Source: three-view drawing plus pictorial views. Frame: mm from the lowest corner of the part. Round coordinates to 2 decimals unless told otherwise and drop trailing zeros. Loops run counter-clockwise (first coordinate to the right, second up) from the corner with the lowest first, then second, coordinate; pieces in that order, holes last. Notation, with made-up numbers: (51, 25) -> (110, 25) arc R27 ccw to (110, 47) -> close; hole circle Ø2 at (54, -13.75). An arc over 180 degrees is marked (long way). One line per question, with ' | ' between items. Start each with the question number.
Q1. Cut plane D-D on x = 5.5. Return loops of the section in (y, z), and give its area (3 significant figures).
Q2. Material intervals for L1, parallel to Y at x = 3, z = 2; L2, parallel to Z at x = 1.1, y = 4.4; L3, parallel to Z at x = 2.55, y = 3.25, sorted ascending.
Q3. Contact query for flat-ended pins moving along their axis: P1, Ø2, axis at y = 3.5, z = 40, coming from the +X side; P2, Ø1, axis at y = 2, z = 5.5, coming from the +X side; P3, Ø2, axis at y = 0.5, z = 12, coming from the -X side. Output: stop coordinate, or through.
Q4. Cut plane B-B on x = 3. Return loops of the section in (y, z).
Q5. Cut plane A-A on z = 18. Return loops of the section in (x, y), and give its area (3 significant figures).
Q6. Cut plane C-C on x = 0.7. Return loops of the section in (y, z).
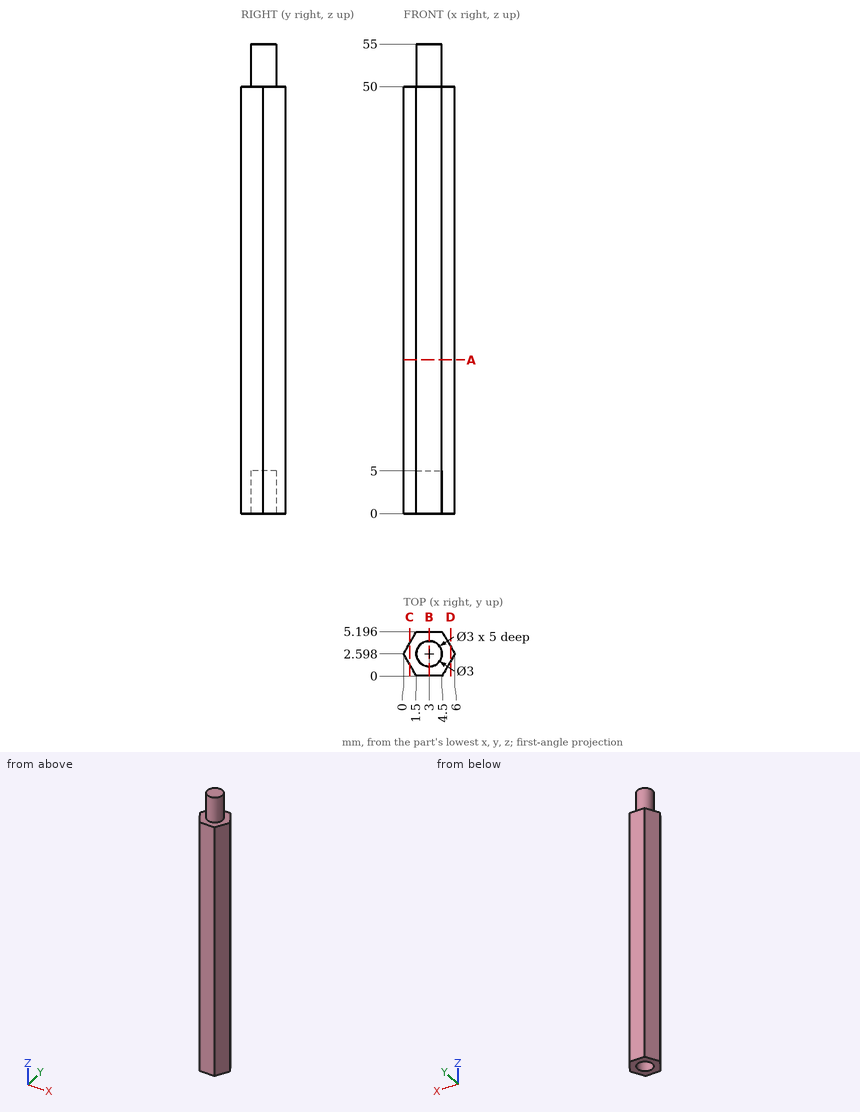
Results:
1) outline: (1.73, 0) -> (3.46, 0) -> (3.46, 50) -> (1.73, 50) -> close | area: 86.6 mm^2
2) L1: 0 to 1.1, 4.1 to 5.2 | L2: 0 to 50 | L3: 5 to 55
3) P1: x = 6 | P2: x = 5.94 | P3: x = 0.63
4) outline: (0, 0) -> (1.1, 0) -> (1.1, 5) -> (4.1, 5) -> (4.1, 0) -> (5.2, 0) -> (5.2, 50) -> (4.1, 50) -> (4.1, 55) -> (1.1, 55) -> (1.1, 50) -> (0, 50) -> close
5) outline: (0, 2.6) -> (1.5, 0) -> (4.5, 0) -> (6, 2.6) -> (4.5, 5.2) -> (1.5, 5.2) -> close | area: 23.4 mm^2
6) outline: (1.39, 0) -> (3.81, 0) -> (3.81, 50) -> (1.39, 50) -> close
